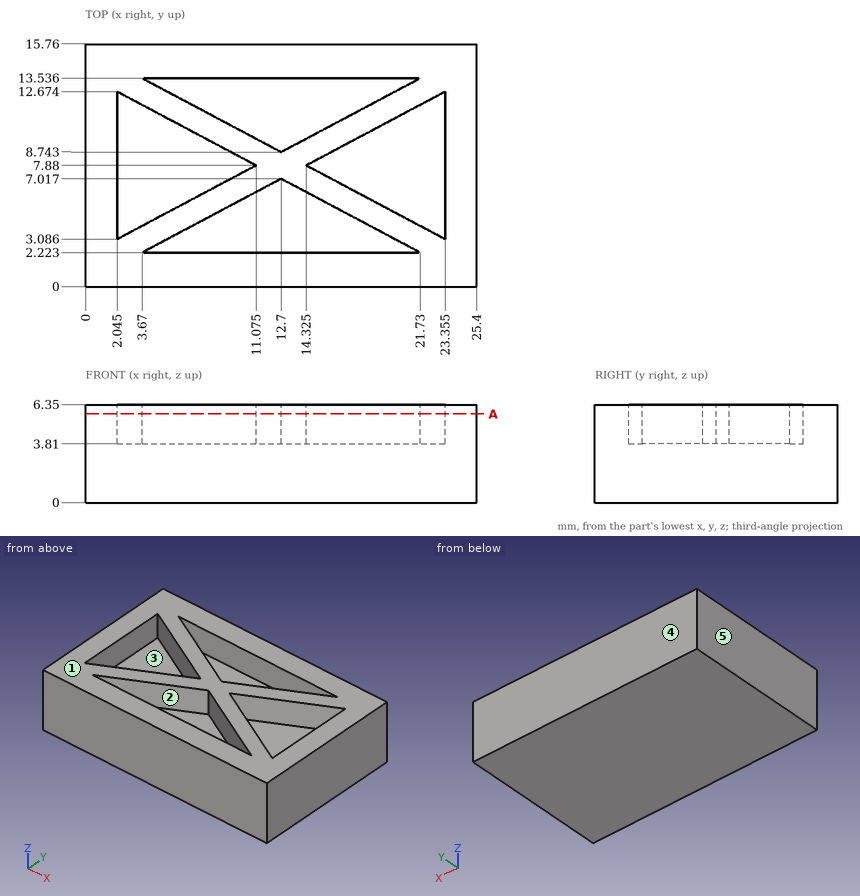
The figure shows three views and two pictorial views of one solid part (mm, origin at its lowest corner). Answer the questions. A direction names the side the tool comes from. Coordinates: 2 decimals unless noted, no trailing zeros. Write each loop counter-clockwise with the first axis right and the second up, starting at its lowest first coordinate (ties: lowest second). Pieces come first, ordered by that corner, then holes. Notation, with made-up numbers: (67.25, -13) -> (94.25, -13) arc R6 cw to (94.25, -5) -> close; hole circle Ø6 at (28.25, 84.25). An arc over 180 degrees is marked (long way). Return JSON: item names as keys, results as strings.
(1) Which of the six approach directions +Z, -Z, +X, -X, +Y, -Y give full straight-line access (tool end or side, diameter ignored) to the marked faces 1 and 2?
Answers below:
{"face 1": "+Z, +X, -X, +Y, -Y", "face 2": "+Z"}
(2) For a pull along X with two mould halves and no side action, classify the marked faces 3, 4 and 5 as pulls with the +X half, pulls with the -X half, needs draft (parallel to the pull), parting line crosses it, or undercut.
Answers below:
{"face 3": "undercut", "face 4": "needs draft", "face 5": "pulls with the -X half"}
(3) The part is cut by section A-A on z = 5.75. Give the vertices of the cut face in (x, y) (1 decimal).
Answers below:
{"outline": "(0, 0) -> (25.4, 0) -> (25.4, 15.8) -> (0, 15.8) -> close; hole (2, 3.1) -> (11.1, 7.9) -> (2, 12.7) -> close; hole (3.7, 2.2) -> (21.7, 2.2) -> (12.7, 7) -> close; hole (3.7, 13.5) -> (12.7, 8.7) -> (21.7, 13.5) -> close; hole (14.3, 7.9) -> (23.4, 3.1) -> (23.4, 12.7) -> close"}
(4) Consider line 1 along X through (y, z) = (4.5, 5.25) (1 decimal); line 2 along Y through (x, z) = (11.5, 5.5) (1 decimal); line 3 along Y through (x, z) = (12.25, 5.5) (1 decimal). Determine where each line is inside the solid, lowest interval first. Write a range as from..to.
Answers below:
{"line 1": "0..2, 4.7..8, 17.4..20.7, 23.4..25.4", "line 2": "0..2.2, 6.4..9.4, 13.5..15.8", "line 3": "0..2.2, 6.8..9, 13.5..15.8"}
